Source: CAD feature listing. Evaluate the final solid. Frame: model axes, mm. Face numbers are marked on the shaded views. Coordinates: 2 decimals unless noted, no trailing zeros. Write each loop counter-clockwise with the first axis right and the second up, starting at its lowest first coordinate (ties: lowest second). Pieces come first, ordered by that corner, then holes. Notation, with made-up numbers: M 25,4 L 32,4 A18 ccw 32,13 Z; hole C 81.5,62 d2. An arc over 180 degrees is marked long. One line per item, written item: value. Start each with the question number.
Item 1: Mould query, pull axis X, two halves, no side actions, for the marked faces 1 and 2. Classes: released by +X, released by -X, zero draft, split by the parting line, or undercut.
Item 2: Cut plane B-B, the plane z = 0. Output: boundary loops of the cut face in (x, y).
Item 3: Cut plane A-A, the plane x = 0. Output: boundary loops of the cut face in (y, z), then the cut area to 3 significant figures.
Item 4: Cut plane D-D, the plane y = 72. Output: boundary loops of the cut face in (x, z).
Item 5: Pin query (flat end, axial travel): P1, Ø4, axis at x = 6.5, z = -0.5, coming from the +Y side; P2, Ø4, axis at y = 32, z = -4, coming from the +X side; P3, Ø5, axis at y = 31.5, z = 4.5, coming from the -X side; P4, Ø4, axis at x = -4, y = 122, coming from the +Z side. Return the tip coordinate at first contact, or that it passes through.
Item 6: Ray query, L1, parallel to Z at x = 0, y = 49; L2, parallel to Y at x = 7.25, z = 0; L3, parallel to Y at x = 0, z = 7.1. Return the intervals inside material, ascending. Write a range as from..to.
Item 7: Cut plane C-C, the plane y = 35. Output: boundary loops of the cut face in (x, z).
```python
from build123d import *

# Parameters (mm, degrees)
SKETCH_1_R               = 8
SKETCH_1_R_2             = 7
EXTRUDE_1_DEPTH          = 150
SKETCH_2_R               = 1.5
CUT_EXTRUDE_1_DEPTH      = 9
CUT_EXTRUDE_1_DEPTH_BACK = 9
SKETCH_4_R               = 1.5
CUT_EXTRUDE_2_DEPTH      = 9.0000001
CUT_EXTRUDE_2_DEPTH_BACK = 9.0000001


with BuildPart() as part:
    # 草图1 → 凸台-拉伸1 (new body)
    with BuildSketch(Plane(origin=(0, 0, 0), x_dir=(1, 0, 0), z_dir=(0, 1, 0))):
        Circle(SKETCH_1_R)
        Circle(SKETCH_1_R_2, mode=Mode.SUBTRACT)
    extrude(amount=EXTRUDE_1_DEPTH)

    # 草图2 → 切除-拉伸1 (cut, two sides)
    with BuildSketch(Plane.XY) as cut_extrude_1_sk:
        with Locations((0, 15)):
            Circle(SKETCH_2_R)
    extrude(amount=CUT_EXTRUDE_1_DEPTH, mode=Mode.SUBTRACT)
    extrude(cut_extrude_1_sk.sketch, amount=-CUT_EXTRUDE_1_DEPTH_BACK, mode=Mode.SUBTRACT)

    # 草图4 → 切除-拉伸2 (cut, two sides)
    with BuildSketch(Plane(origin=(0, 0, 0), x_dir=(0, 0, -1), z_dir=(1, 0, 0))) as cut_extrude_2_sk:
        with Locations((0, 35)):
            Circle(SKETCH_4_R)
    extrude(amount=CUT_EXTRUDE_2_DEPTH, mode=Mode.SUBTRACT)
    extrude(cut_extrude_2_sk.sketch, amount=-CUT_EXTRUDE_2_DEPTH_BACK, mode=Mode.SUBTRACT)


solid = part.part
```
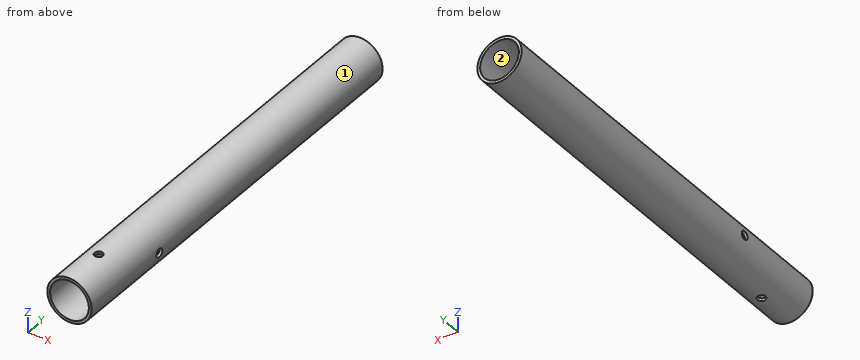
From the geometry:
1. face 1: split by the parting line
1. face 2: undercut
2. outline: M -8,0 L -7,0 L -7,33.5 L -8,33.5 Z; M -8,36.5 L -7,36.5 L -7,150 L -8,150 Z; M 7,0 L 8,0 L 8,33.5 L 7,33.5 Z; M 7,36.5 L 8,36.5 L 8,150 L 7,150 Z
3. outline: M 0,-8 L 13.5,-8 L 13.5,-7 L 0,-7 Z; M 0,7 L 13.5,7 L 13.5,8 L 0,8 Z; M 16.5,-8 L 150,-8 L 150,-7 L 16.5,-7 Z; M 16.5,7 L 150,7 L 150,8 L 16.5,8 Z
3. area: 294 mm²
4. outline: C 0,0 d16; hole C 0,0 d14
5. P1: stops at y = 150
5. P2: stops at x = 7.75
5. P3: stops at x = -7.75
5. P4: stops at z = 7.75
6. L1: z = -8..-7, 7..8
6. L2: y = 0..33.5, 36.5..150
6. L3: y = 0..13.5, 16.5..150
7. outline: M -7.86,-1.5 A8 ccw 7.86,-1.5 L 6.84,-1.5 A7 cw -6.84,-1.5 Z; M -7.86,1.5 L -6.84,1.5 A7 cw 6.84,1.5 L 7.86,1.5 A8 ccw Z
